Verification items for the finished model (mm, model axes). A direction names the side the tool comes from. Round coordinates to 2 decimals unless told otherwise and drop trailing zeros. Answer as a JSON object with one key per item and string values.
```python
from build123d import *

# Parameters (mm, degrees)
SKETCH3_R   = 20
SKETCH3_R_2 = 15


with BuildPart() as part:
    # Sweep1: sweep along a path in Sketch2
    with BuildLine(Plane.XY) as sweep1_path:
        Line((0, 0), (70.636050153, 0))
        ThreePointArc((70.636050153, 0), (97.010850822, -6.107793795), (118.015923362, -23.187670345))
        Line((118.015923362, -23.187670345), (122.240253581, -28.624659311))
        ThreePointArc((122.240253581, -28.624659311), (164.250398662, -62.78441241), (217, -75))
        Line((217, -75), (933, -75))
        ThreePointArc((933, -75), (985.749601338, -62.78441241), (1027.759746419, -28.624659311))
        Line((1027.759746419, -28.624659311), (1031.984076638, -23.187670345))
        ThreePointArc((1031.984076638, -23.187670345), (1052.989149178, -6.107793795), (1079.363949847, 0))
        Line((1079.363949847, 0), (1150, 0))
    # Sketch3 → Sweep1 (sweep)
    with BuildSketch(Plane(origin=(0, 0, 0), x_dir=(0, 0, -1), z_dir=(1, 0, 0))):
        Circle(SKETCH3_R)
        Circle(SKETCH3_R_2, mode=Mode.SUBTRACT)
    sweep(path=sweep1_path.line)


solid = part.part
```
1. Go/stop test with flat-tipped pins: pin 1 (6 mm diameter, centred on x = 599.5, z = 1, fed in from +Y); pin 2 (8 mm diameter, centred on x = 433, z = 9.5, fed in from -Y); pin 3 (3 mm diameter, centred on x = 1032, y = -38, fed in from -Z). Record where each tip stops, or that it passes through.
Completed:
{"pin 1": "stops at y = -55", "pin 2": "stops at y = -94.23", "pin 3": "stops at z = -18.46"}
2. Access from +Z, -Z, +X, -X, +Y, -Y to the whole of each face (thin tool, end or side, straight path). Record for faces 4 (the face through (1150, -15, 3)), 5 (the face through (580.012, -89.643, 3.252)), 6 (the face through (35.812, -19.524, 4.336)), 7 (the face through (1115.176, 0.66, 14.985)).
Completed:
{"face 4": "+Z, -Z, +X, +Y, -Y", "face 5": "none", "face 6": "-X", "face 7": "+X"}
3. Mould release check, pull along Y, two halves, no side actions. Record for faces 1 (the face through (580.012, -94.524, 4.336)), 2 (the face through (0, -15, 3)), 3 (the face through (108.594, -34.928, 3.252)): released by +Y, released by -Y, zero draft, split by the parting line, or undercut.
Completed:
{"face 1": "split by the parting line", "face 2": "zero draft", "face 3": "undercut"}
4. Material ranges on probe 1 along Y at (x, z) = (741.5, 0); probe 2 along X at (y, z) = (-17, 8); probe 3 along X at (y, z) = (-6, -5), recorded low to high. Write a range as from..to.
Completed:
{"probe 1": "y = -95..-90, -60..-55", "probe 2": "x = 0..90.37, 129.28..136.42, 1013.58..1020.72, 1059.63..1150", "probe 3": "x = 121.44..128.8, 1021.2..1028.56"}
